```python
from build123d import *

# Parameters (mm, degrees)
BOSS_EXTRUDE1_DEPTH                            = 25.4
SKETCH5_R                                      = 3.96875
CUT_EXTRUDE2_DEPTH                             = 4.175
CSK_FOR_2_FLAT_HEAD_MACHINE_SCREW1_D           = 2.4384
CSK_FOR_2_FLAT_HEAD_MACHINE_SCREW1_DEPTH       = 3.175
CSK_FOR_2_FLAT_HEAD_MACHINE_SCREW1_CSINK_D     = 4.3688
CSK_FOR_2_FLAT_HEAD_MACHINE_SCREW1_CSINK_ANGLE = 82
SKETCH9_W                                      = 2.54
SKETCH9_H                                      = 25.4
CUT_EXTRUDE3_DEPTH                             = 4.175
FILLET1_R                                      = 2.54
SKETCH10_W                                     = 0.254
SKETCH10_H                                     = 25.4
CUT_EXTRUDE4_DEPTH                             = 26.4


with BuildPart() as part:
    # Sketch1 → Boss-Extrude1 (new body)
    with BuildSketch(Plane.XY):
        Polygon((0, 0), (25.4, 0), (25.4, 3.175), (3.175, 3.175), (3.175, 25.4), (0, 25.4), align=None)
    extrude(amount=BOSS_EXTRUDE1_DEPTH)

    # Sketch5 → Cut-Extrude2 (cut, through all)
    with BuildSketch(Plane(origin=(3.175, 0, 0), x_dir=(0, 0, -1), z_dir=(1, 0, 0))):
        with Locations((-12.7, 12.7)):
            Circle(SKETCH5_R)
    extrude(amount=-CUT_EXTRUDE2_DEPTH, mode=Mode.SUBTRACT)

    # CSK for #2 Flat Head Machine Screw1
    with Locations(Plane(origin=(0, 3.175, 0), x_dir=(1, 0, 0), z_dir=(0, 1, 0))):
        with Locations((14.2875, -19.05), (14.2875, -6.35)):
            CounterSinkHole(CSK_FOR_2_FLAT_HEAD_MACHINE_SCREW1_D / 2, CSK_FOR_2_FLAT_HEAD_MACHINE_SCREW1_CSINK_D / 2, depth=CSK_FOR_2_FLAT_HEAD_MACHINE_SCREW1_DEPTH, counter_sink_angle=CSK_FOR_2_FLAT_HEAD_MACHINE_SCREW1_CSINK_ANGLE)

    # Sketch9 → Cut-Extrude3 (cut, through all)
    with BuildSketch(Plane(origin=(0, 3.175, 0), x_dir=(1, 0, 0), z_dir=(0, 1, 0))):
        with Locations((24.13, -12.7)):
            Rectangle(SKETCH9_W, SKETCH9_H)
    extrude(amount=-CUT_EXTRUDE3_DEPTH, mode=Mode.SUBTRACT)

    # Fillet1
    fillet1_edges = [part.edges().sort_by_distance(p)[0] for p in [
        (3.175, 3.175, 12.7),
    ]]
    fillet(fillet1_edges, radius=FILLET1_R)

    # Sketch10 → Cut-Extrude4 (cut, through all)
    with BuildSketch(Plane(origin=(0, 25.4, 0), x_dir=(1, 0, 0), z_dir=(0, 1, 0))):
        with Locations((0.127, -12.7)):
            Rectangle(SKETCH10_W, SKETCH10_H)
    extrude(amount=-CUT_EXTRUDE4_DEPTH, mode=Mode.SUBTRACT)


solid = part.part
```
Part model, mm, in its own coordinate system. A direction names the side the tool comes from. Give positions to 0.01 mm unless a question says otherwise; leave off trailing zeros. Order: outer loops, then holes, each group sorted by start corner. A loop starts at its lowest first (then second) coordinate and runs counter-clockwise, first axis right, second up. Notation, with made-up numbers: (-25, 47.25) - (-1, 47.25) arc R3 cw to (-1, 51.25) - close; hole circle Ø9 at (58, 88). An arc over 180 degrees is marked (long way). Use one line per item in the form item = value.
Item 1: Pin check, flat tips, straight feed: pin 1 Ø10 at (y, z) = (20.5, 17) entering from +X (3 decimals); pin 2 Ø2 at (x, z) = (14.5, 6.5) entering from +Y; pin 3 Ø12 at (x, z) = (12.5, 15.5) entering from +Y (3 decimals). Stop position of each tip, or through.
Solution:
pin_1 = 3.175
pin_2 = 2.11
pin_3 = 3.175
Item 2: Slice it at D-D on x = 17.5. Give the cut face in (y, z) (3 decimals), and give its area (3 significant figures).
Solution:
outline = (0, 0) - (3.175, 0) - (3.175, 25.4) - (0, 25.4) - close
area = 80.6 mm2
Item 3: Slice it at A-A on z = 12.7. Give the cut face in (x, y) (3 decimals).
Solution:
outline = (0.254, 0) - (22.86, 0) - (22.86, 3.175) - (5.715, 3.175) arc R2.54 cw to (3.175, 5.715) - (3.175, 8.731) - (0.254, 8.731) - close; (0.254, 16.669) - (3.175, 16.669) - (3.175, 25.4) - (0.254, 25.4) - close
Item 4: Slice it at B-B on y = 12.7. Give the cut face in (x, z) (3 decimals), and give its area (3 significant figures).
Solution:
outline = (0.254, 0) - (3.175, 0) - (3.175, 8.731) - (0.254, 8.731) - close; (0.254, 16.669) - (3.175, 16.669) - (3.175, 25.4) - (0.254, 25.4) - close
area = 51.0 mm2
Item 5: Two-plate mould, pull along Z, no slides. Class faces 1 (the face through (15.506, 1.018, 6.296)), 2 (the face through (3, 8, 0)), 3 (the face through (14, 3.175, 13)), 4 (the face through (14.55, 1.02, 20.24)): released by +Z, released by -Z, zero draft, split by the parting line, or undercut.
Solution:
face_1 = undercut
face_2 = released by -Z
face_3 = zero draft
face_4 = undercut
Item 6: Probe probe 1 along Y at (x, z) = (2.1, 12.7); probe 2 along Z at (x, y) = (3, 12.5); probe 3 along X at (y, z) = (6.25, 6.5) (3 decimals). List the from-to ranges inside material, lowest first. Write a range as from..to.
Solution:
probe_1 = 0..8.73, 16.67..25.4
probe_2 = 0..8.74, 16.66..25.4
probe_3 = 0.254..3.175
Item 7: Slice it at C-C on z = 2.75. Give the cut face in (x, y) (3 decimals), and give its area (3 significant figures).
Solution:
outline = (0.254, 0) - (22.86, 0) - (22.86, 3.175) - (5.715, 3.175) arc R2.54 cw to (3.175, 5.715) - (3.175, 25.4) - (0.254, 25.4) - close
area = 138 mm2
Item 8: Which spindle directions (+Z, -Z, +X, -X, +Y, -Y) get a long thin tool onto all of the face, cutting with end or side? Do faces 5 (the face through (3.175, 18, 13)), 6 (the face through (1.735, 11.18, 9.034)). Say none if no direction does.
Solution:
face_5 = +Z, -Z, +X, +Y
face_6 = +X, -X
